Part model, mm, in its own coordinate system. Face numbers are marked on the shaded views. A direction names the side the tool comes from. Coordinates: 2 decimals unless noted, no trailing zeros. Write each loop counter-clockwise with the first axis right and the second up, starting at its lowest first coordinate (ties: lowest second). Pieces come first, ordered by that corner, then holes. Notation, with made-up numbers: (62.5, -4.75) - (89.5, -4.75) arc R34 cw to (89.5, 34.25) - close; hole circle Ø3 at (86, 75). An arc over 180 degrees is marked (long way). Use a Markdown table: item, result.
```python
from build123d import *

# Parameters (mm, degrees)
SKETCH1_R           = 57.15
BOSS_EXTRUDE1_DEPTH = 190.5
CUT_EXTRUDE1_START  = -190.5
CUT_EXTRUDE1_DEPTH  = 190.5
SHELL2_START        = 12.7
SHELL2_DEPTH        = 177.8


# Read off the part's stored shape, not the designer's step: Shell2
with BuildPart() as part:
    # Sketch1 → Boss-Extrude1 (new body)
    with BuildSketch(Plane(origin=(0, 0, 0), x_dir=(1, 0, 0), z_dir=(0, 1, 0))):
        with Locations(Location((0, 0, 0), (0, 0, 270))):
            Circle(SKETCH1_R)
    extrude(amount=BOSS_EXTRUDE1_DEPTH)

    # Sketch2 → Cut-Extrude1 (cut)
    with BuildSketch(Plane(origin=(0, 190.5, 0), x_dir=(1, 0, 0), z_dir=(0, 1, 0)).offset(CUT_EXTRUDE1_START)):
        with BuildLine():
            Line((42.597094971, 38.1), (42.597094971, -38.1))
            ThreePointArc((42.597094971, -38.1), (53.387950315, -20.392382431), (57.15, 0))
            ThreePointArc((57.15, 0), (53.387950315, 20.392382431), (42.597094971, 38.1))
        make_face()
    extrude(amount=CUT_EXTRUDE1_DEPTH, mode=Mode.SUBTRACT)

    # Shell2 outline → Shell2 (cut)
    with BuildSketch(Plane(origin=(0, 0, 0), x_dir=(1, 0, 0), z_dir=(0, 1, 0)).offset(SHELL2_START)):
        with BuildLine():
            ThreePointArc((17.197094971, 51.831573626), (-54.61, 0), (17.197094971, -51.831573626))
            Line((17.197094971, -51.831573626), (17.197094971, 51.831573626))
        make_face()
    extrude(amount=SHELL2_DEPTH, mode=Mode.SUBTRACT)


solid = part.part
```
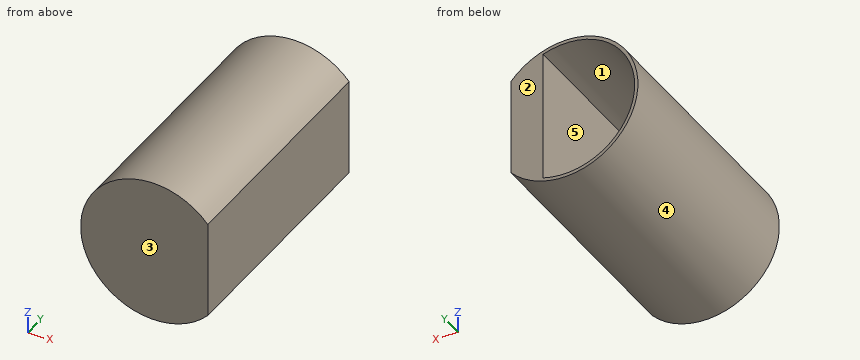
Item 1: Band-saw the part on C-C, the plane y = 179.5. Give the cut face in (x, z), then the cut area to 3 significant figures.
From the geometry:
| item | result |
|---|---|
| outline | (42.6, -38.1) - (42.6, 38.1) arc R57.15 ccw (long way) to start; hole (17.2, -51.83) - (17.2, 51.83) arc R54.61 ccw (long way) to start |
| area | 2,970 mm^2 |
Item 2: Two-plate mould, pull along Z, no slides. Class the marked faces 3, 4 and 5: pulls with the +Z half, pulls with the -Z half, needs draft (parallel to the pull), parting line crosses it, or undercut.
From the geometry:
| item | result |
|---|---|
| face 3 | needs draft |
| face 4 | parting line crosses it |
| face 5 | undercut |
Item 3: Which spindle directions (+Z, -Z, +X, -X, +Y, -Y) get a long thin tool onto all of the face, cutting with end or side? Do the marked faces 1 and 2. Say none if no direction does.
From the geometry:
| item | result |
|---|---|
| face 1 | +Y |
| face 2 | +Z, -Z, +X, -X, +Y |
Item 4: Band-saw the part on A-A, the plane x = 0. Give the cut face in (y, z), then the cut area to 3 significant figures.
From the geometry:
| item | result |
|---|---|
| outline | (0, -57.15) - (190.5, -57.15) - (190.5, -54.61) - (12.7, -54.61) - (12.7, 54.61) - (190.5, 54.61) - (190.5, 57.15) - (0, 57.15) - close |
| area | 2,350 mm^2 |
Item 5: Band-saw the part on B-B, the plane z = 0. Give the cut face in (x, y), then the cut area to 3 significant figures.
From the geometry:
| item | result |
|---|---|
| outline | (-57.15, 0) - (42.6, 0) - (42.6, 190.5) - (17.2, 190.5) - (17.2, 12.7) - (-54.61, 12.7) - (-54.61, 190.5) - (-57.15, 190.5) - close |
| area | 6,230 mm^2 |
Item 6: Drill centre lines: probe 1 along X at (y, z) = (115, 0); probe 2 along Y at (x, z) = (12, 3); probe 3 along X at (y, z) = (176, -38.5). Where is each one in solid material? Low to high.
From the geometry:
| item | result |
|---|---|
| probe 1 | -57.15 to -54.61, 17.2 to 42.6 |
| probe 2 | 0 to 12.7 |
| probe 3 | -42.24 to -38.73, 17.2 to 42.24 |
Item 7: Drop flat-ended pins along their axis: P1, Ø3, axis at x = -16, z = -13.5, coming from the +Y side; P2, Ø12, axis at x = 10, y = 55, coming from the +Z side; P3, Ø2, axis at x = 27.5, y = 22, coming from the -Z side. Give the stop position or say it passes through.
From the geometry:
| item | result |
|---|---|
| P1 | y = 12.7 |
| P2 | z = 57.01 |
| P3 | z = -50.63 |
